Design review of the part shown in the three views and the two pictorial views. Dimensions are in mm from the part's minimum x, y and z. A direction names the side the tool comes from. Round coordinates to 2 decimals unless told otherwise and drop trailing zeros. Order: outer loops, then holes, each group sorted by start corner. A loop starts at its lowest first (then second) coordinate and runs counter-clockwise, first axis right, second up. Notation, with made-up numbers: (33, 14.5) - (53, 14.5) arc R19 ccw to (53, 42.5) - close; hole circle Ø4 at (80.25, 55). An arc over 180 degrees is marked (long way). One line per question, with ' | ' between items. Start each with the question number.
Item 1: Insertion check: pin 1 Ø10 at (x, z) = (12, 3.5) entering from +Y. The pin has a flat end and moves straight along its axis. Give the tip position at first contact, or say it passes through.
Item 2: For L1, parallel to Z at x = 15, y = 24.5; L2, parallel to Z at x = 15, y = 26.5; L3, parallel to Y at x = 25.25, z = 6.25, list the stretches that pass through material, from the lowest coordinate up. Write a range as [from, to].
Item 3: Add section B-B on y = 27.75. State the section outline as (x, z) points, and give its area (3 significant figures).
Item 4: Add section D-D on x = 20.5. State the section outline as (y, z) points, and give its area (3 significant figures).
Item 5: Add section C-C on z = 15. State the section outline as (x, y) points, and give its area (3 significant figures).
Item 6: Tool access review of the marked faces 5 and 6: name each direction out of +Z, -Z, +X, -X, +Y, -Y from which nothing blocks a thin tool from reaching the whole face with its end or side.
Item 7: Draft analysis for pull direction X (two halves, no side actions). For the marked faces 1, 2, 3 and 4, state which applies: +X half, -X half, draft (parallel to the pull), parting line (faces both ways), or undercut.
Item 8: Add section A-A on x = 15. State the section outline as (y, z) points.
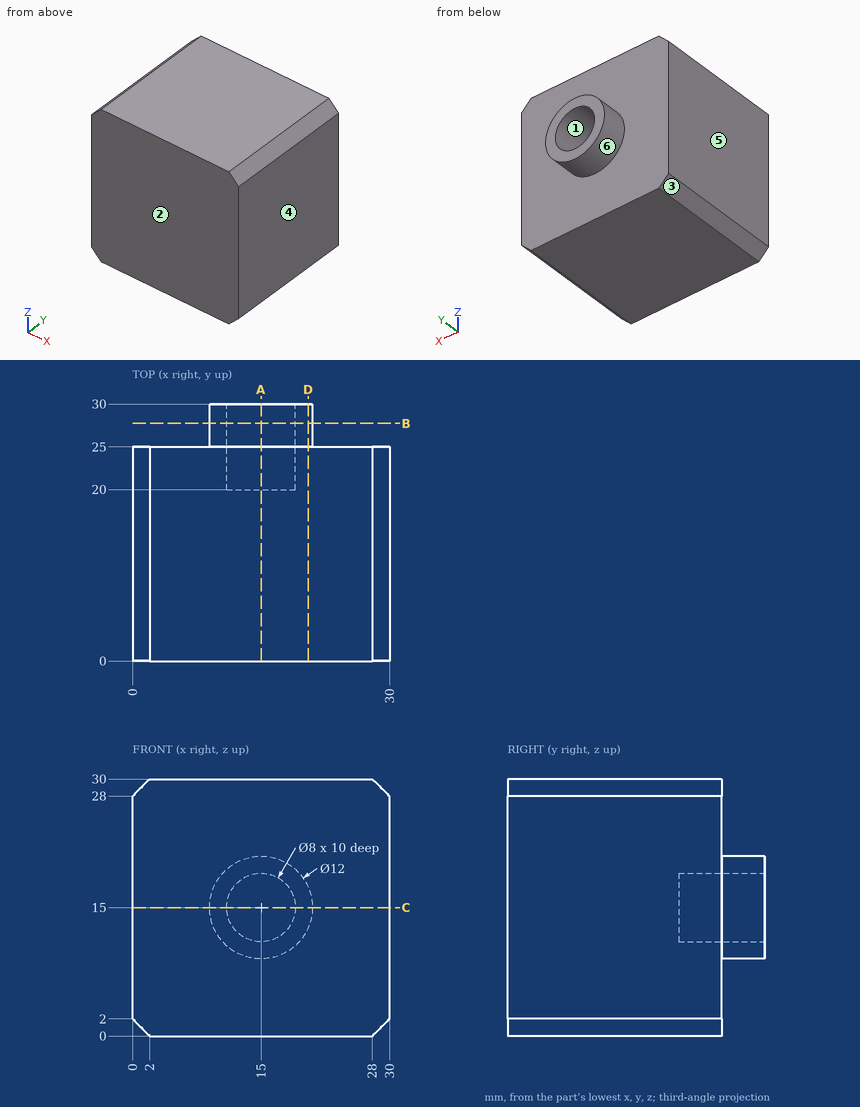
Determined:
1) pin 1: y = 25
2) L1: [0, 11], [19, 30] | L2: [9, 11], [19, 21] | L3: [0, 25]
3) outline: circle Ø12 at (15, 15); hole circle Ø8 at (15, 15) | area: 62.8 mm2
4) outline: (0, 0) - (25, 0) - (25, 12.6) - (30, 12.6) - (30, 17.4) - (25, 17.4) - (25, 30) - (0, 30) - close | area: 774 mm2
5) outline: (0, 0) - (30, 0) - (30, 25) - (21, 25) - (21, 30) - (19, 30) - (19, 20) - (11, 20) - (11, 30) - (9, 30) - (9, 25) - (0, 25) - close | area: 730 mm2
6) face 5: +Z, -Z, -X, +Y, -Y | face 6: +Y
7) face 1: undercut | face 2: draft | face 3: -X half | face 4: +X half
8) outline: (0, 0) - (25, 0) - (25, 9) - (30, 9) - (30, 11) - (20, 11) - (20, 19) - (30, 19) - (30, 21) - (25, 21) - (25, 30) - (0, 30) - close
